Autodesk Inventor part; units mm, degrees
ref_plane "YZ Plane" through (0, 0, 0) normal (1, 0, 0) x (0, 1, 0)
ref_plane "XZ Plane" through (0, 0, 0) normal (0, 1, 0) x (-1, 0, 0)
ref_plane "XY Plane" through (0, 0, 0) normal (0, 0, 1) x (1, 0, 0)
sketch "Sketch1" plane through (0, 0, 0) normal (0, 0, 1) x (1, 0, 0)
  circle A0 centre (0, 0) radius 2
  circle A1 centre (0, 0) radius 1
  dimension "d0" = 2
  dimension "d1" = 4
extrude "Extrusion1" add sketch "Sketch1" along normal blind 35
sketch "Sketch2" plane through (0, 0, 0) normal (1, 0, 0) x (0, 1, 0)
  line L0 (-2, 35) -> (2, 35)
  line L1 (-2, 35) -> (2, 35)
  line L2 (-2, 0) -> (2, 0)
  line L3 (1, 0) -> (1, 35)
  line L4 (2, 0) -> (2, 35)
  line L5 (-2, 0) -> (-2, 35)
  line L6 (0, -7.8082) -> (0, 46.8491)
  line L7 (-1, 0) -> (-1, 35)
  spline S0 degree 4 poles (2.5, 37.1511) (2.4385, 36.2785) (2.4715, 36.4932) (2, 35.6037) (2, 35) knots 0 0 0 0 0 1 1 1 1 1
  line L8 (1.85, 39) -> (2.5, 39)
  line L9 (2.5455, 37.7966) -> (2.4545, 36.5056) construction
  arc A0 (2.5379, 37.6674) -> (2.4651, 36.6346) centre (93.2146, 30.7544) ccw construction
  line L10 (1, 35) -> (2, 35)
  spline S1 degree 4 poles (1.85, 39) (1.85, 38.3805) (1.9584, 36.9535) (1.8064, 36.2993) (1, 35.4823) (1, 35) knots 0 0 0 0 0 0.518957 1 1 1 1 1
  line L11 (1.85, 39) -> (1.85, 33.7099)
  spline S2 degree 1 poles (2.5, 39) (2.5, 37.1511) knots 0 0 1 1
  point P0 (0, 0)
  point P1 (2.85, 39)
  point P2 (1.85, 37.1511)
  point P3 (1.4925, 36.0895)
  dimension "d6" = 1
  dimension "d9" = 4
  dimension "d10" = 0.65
  dimension "d11" = 2.5
revolve "Revolution1" add sketch "Sketch2" angle 360 about axis through (0, 0, -10) along (0, 0, 1) contours S1 L11 L0 | L11 S1 L8 S2 S0 L0
sketch "Sketch3" plane through (0, 0, 0) normal (0, 0, -1) x (-1, 0, 0)
  circle A0 centre (0, 0) radius 2
  circle A1 centre (0, 0) radius 1
  circle A2 centre (0, 0) radius 2
extrude "Extrusion2" cut sketch "Sketch3" against normal blind 7.215
equation "\"d0\" = GuideTubingID"
equation "\"d1\" = GuideTubingOD"
equation "\"d10\" = 0.65 * d6"
equation "\"baseOD\" = 23"
equation "\"baseInitD\" = 4"
equation "\"baseTh0\" = 48.463041deg"
equation "\"baseTh1\" = 23.073918deg"
equation "\"topD\" = 14"
equation "\"topInitD\" = 4"
equation "\"topTh0\" = 16.60155deg"
equation "\"topTh1\" = 86.796901deg"
equation "\"dFlexure\" = 0.38"
equation "\"lFlexure\" = 1.5"
equation "\"lFlexureOffset\" = 1.95"
equation "\"dMotor\" = 1.44"
equation "\"lMotor\" = 22.35"
equation "\"topH\" = 21.66629"
equation "\"springBaseD\" = 8"
equation "\"springTopD\" = 8"
equation "\"springInitL\" = 12.7"
equation "\"springLset\" = 3.5"
equation "\"springDeform\" = 18.16629"
equation "\"springL\" = 30.86629"
equation "\"springLO\" = 33.86629"
equation "\"springUnderCut\" = 9.2"
equation "\"dM1X\" = 6.73587"
equation "\"dM1Y\" = 2.34012"
equation "\"dM2X\" = -1.34133"
equation "\"dM2Y\" = 7.00349"
equation "\"dM1Xt\" = 6.59227"
equation "\"dM1Yt\" = -0.43704"
equation "\"dM2Xt\" = -3.67462"
equation "\"dM2Yt\" = 5.49055"
equation "\"GuideRod\" = 2"
equation "\"GuideTubingOD\" = 4"
equation "\"GuideTubingID\" = 2"
equation "\"CSpringOD\" = 5.537"
equation "\"CSpringCD\" = 0.254"
equation "\"CSpringID\" = 5.029"
equation "\"d7\" = d6"
properties part number "Spring Guide Tube" material "Viton"
Geometry check sheet. Reference: the model listing, model coordinates, mm. Round coordinates to 2 decimals unless told otherwise and drop trailing zeros. Order: outer loops, then holes, each group sorted by start corner. A loop starts at its lowest first (then second) coordinate and runs counter-clockwise, first axis right, second up. Notation, with made-up numbers: (-31.75, 73) - (2.25, 73) arc R20 ccw to (2.25, 112) - close; hole circle Ø7 at (-26, 72.25). An arc over 180 degrees is marked (long way). Use a Markdown table: item, result. Add a question column.
1) Mould release check, pull along Y, two halves, no side actions. Record for faces 1 (the cylindrical face through (0, 1, 21)), 2 (the cylindrical face through (0, 2, 21)), 3 (the flat face through (-1, -1, 7.215)): released by +Y, released by -Y, zero draft, split by the parting line, or undercut.
2) Gauge pin test, flat ends, axial feed: P1, Ø2, axis at x = 0, z = 17.5, coming from the -Y side; P2, Ø2, axis at y = 0, z = 25, coming from the +X side; P3, Ø1.6, axis at x = 0, y = 0, coming from the -Z side; P4, Ø1, axis at x = -0.5, z = 26, coming from the +Y side. Record the tip position at first contact, or that the pin passes through.
3) Thickness scan on line 1 along Y through (x, z) = (0, 20.25); line 2 along X through (y, z) = (-0.6, 16). Record the ranges inside material, lowest first.
4) Section check A-A (z = 24.5). Record the cut outline in (x, y).
Established:
| question | item | result |
|---|---|---|
| 1 | face 1 | undercut |
| 1 | face 2 | split by the parting line |
| 1 | face 3 | zero draft |
| 2 | P1 | y = -2 |
| 2 | P2 | x = 2 |
| 2 | P3 | through |
| 2 | P4 | y = 2 |
| 3 | line 1 | -2 to -1, 1 to 2 |
| 3 | line 2 | -1.91 to -0.8, 0.8 to 1.91 |
| 4 | outline | circle Ø4 at (0, 0); hole circle Ø2 at (0, 0) |
